from build123d import *

# Parameters (mm, degrees)
ESBO_O1_R                = 5.25
ESBO_O1_R_2              = 3.225
ESBO_O1_R_3              = 2.5
RESSALTO_EXTRUS_O1_DEPTH = 5


with BuildPart() as part:
    # Esboço1 → Ressalto-extrusão1 (new body)
    with BuildSketch(Plane.XY):
        with BuildLine():
            Line((0.238095238, -10.714285714), (31.238095238, -10.714285714))
            ThreePointArc((31.238095238, -10.714285714), (34.066522363, -11.88585859), (35.238095238, -14.714285714))
            Line((35.238095238, -14.714285714), (35.238095238, -18.714285714))
            ThreePointArc((35.238095238, -18.714285714), (35.823881676, -20.128499277), (37.238095238, -20.714285714))
            Line((37.238095238, -20.714285714), (53.238095238, -20.714285714))
            ThreePointArc((53.238095238, -20.714285714), (54.6523088, -20.128499277), (55.238095238, -18.714285714))
            Line((55.238095238, -18.714285714), (55.238095238, -2.714285714))
            ThreePointArc((55.238095238, -2.714285714), (54.6523088, -1.300072152), (53.238095238, -0.714285714))
            Line((53.238095238, -0.714285714), (31.847818571, -0.714285714))
            ThreePointArc((31.847818571, -0.714285714), (14.124879647, 4.104636838), (1.282253299, 17.234432234))
            ThreePointArc((1.282253299, 17.234432234), (-0.185475427, 18.73498028), (-2.210954161, 19.285714286))
            Line((-2.210954161, 19.285714286), (-17.761904762, 19.285714286))
            ThreePointArc((-17.761904762, 19.285714286), (-19.176118324, 19.871500723), (-19.761904762, 21.285714286))
            Line((-19.761904762, 21.285714286), (-19.761904762, 27.285714286))
            ThreePointArc((-19.761904762, 27.285714286), (-20.3476912, 28.699927848), (-21.761904762, 29.285714286))
            Line((-21.761904762, 29.285714286), (-37.761904762, 29.285714286))
            ThreePointArc((-37.761904762, 29.285714286), (-39.176118324, 28.699927848), (-39.761904762, 27.285714286))
            Line((-39.761904762, 27.285714286), (-39.761904762, -18.714285714))
            ThreePointArc((-39.761904762, -18.714285714), (-39.176118324, -20.128499277), (-37.761904762, -20.714285714))
            Line((-37.761904762, -20.714285714), (-21.761904762, -20.714285714))
            ThreePointArc((-21.761904762, -20.714285714), (-20.3476912, -20.128499277), (-19.761904762, -18.714285714))
            Line((-19.761904762, -18.714285714), (-19.761904762, -14.714285714))
            ThreePointArc((-19.761904762, -14.714285714), (-18.590331887, -11.88585859), (-15.761904762, -10.714285714))
            Line((-15.761904762, -10.714285714), (0.238095238, -10.714285714))
        make_face()
        with Locations((-29.761904762, -13.571428571)):
            Circle(ESBO_O1_R, mode=Mode.SUBTRACT)
        with Locations((-29.761904762, 21.904761905)):
            Circle(ESBO_O1_R_2, mode=Mode.SUBTRACT)
        with Locations((-4.761904762, 4.285714286)):
            Circle(ESBO_O1_R_3, mode=Mode.SUBTRACT)
        with Locations((45.476190476, -10.714285714)):
            Circle(ESBO_O1_R, mode=Mode.SUBTRACT)
    extrude(amount=RESSALTO_EXTRUS_O1_DEPTH)


solid = part.part
Could you check a few things on this model? Use its own coordinates, in mm. A direction names the side the tool comes from. Give positions to 0.01 mm unless a question says otherwise; leave off trailing zeros. Loops run counter-clockwise (first coordinate to the right, second up) from the corner with the lowest first, then second, coordinate; pieces in that order, holes last. Notation, with made-up numbers: (11.25, 16) -> (18.25, 16) arc R13 cw to (18.25, 31) -> close; hole circle Ø4 at (86.5, 2). An arc over 180 degrees is marked (long way). Return JSON: item names as keys, results as strings.
Item 1: I need wall thicknesses on L1, parallel to X at y = -18, z = 3; L2, parallel to Y at x = 45, z = 4.15; L3, parallel to X at y = -17.5, z = 3.15. Which ranges of each line are inside material? Lowest first, please. Write a range as from..to.
Geometry results:
{"L1": "x = -39.76..-32.58, -26.94..-19.76, 35.24..55.24", "L2": "y = -20.71..-15.94, -5.49..-0.71", "L3": "x = -39.76..-33.24, -26.28..-19.76, 35.24..55.24"}
Item 2: I'm going to push flat-ended pins straight in: pin 1 (2.5 mm diameter, centred on y = 25, z = 3.5, fed in from +X); pin 2 (1.5 mm diameter, centred on x = 41, z = 1.5, fed in from +Y); pin 3 (2.5 mm diameter, centred on x = -12, z = 1.5, fed in from +Y). Where does each tip first touch, or does it pass through?
Geometry results:
{"pin 1": "stops at x = -19.76", "pin 2": "stops at y = -0.71", "pin 3": "stops at y = 19.29"}
Item 3: If we section it at A-A on x = 43: List the corners of the cut face in (y, z) for me.
Geometry results:
{"outline": "(-20.71, 0) -> (-15.34, 0) -> (-15.34, 5) -> (-20.71, 5) -> close; (-6.08, 0) -> (-0.71, 0) -> (-0.71, 5) -> (-6.08, 5) -> close"}
Item 4: Which directions (+Z, -Z, +X, -X, +Y, -Y) give clear straight access to the entire face, cutting with the end or side of a thin tool? Please do faces 1 (the cylindrical face through (35.808, -20.113, 2.465)), 2 (the flat face through (-39.762, 5, 2)), 3 (the flat face through (43, -0.714, 2)).
Geometry results:
{"face 1": "+Z, -Z, -Y", "face 2": "+Z, -Z, -X, +Y, -Y", "face 3": "+Z, -Z, +X, +Y"}
Item 5: If we section it at D-D on x = -12.5: List the corners of the cut face in (y, z) for me, plus the area to 3 significant figures.
Geometry results:
{"outline": "(-10.71, 0) -> (19.29, 0) -> (19.29, 5) -> (-10.71, 5) -> close", "area": "150 mm²"}
Item 6: If we section it at B-B on y = 24: List the corners of the cut face in (x, z) for me, plus the area to 3 significant figures.
Geometry results:
{"outline": "(-39.76, 0) -> (-32.21, 0) -> (-32.21, 5) -> (-39.76, 5) -> close; (-27.31, 0) -> (-19.76, 0) -> (-19.76, 5) -> (-27.31, 5) -> close", "area": "75.5 mm²"}
Item 7: We'd pull the mould along X, two halves only. Please class faces 4 (the cylindrical face through (-39.192, -20.113, 2.465)), 5 (the cylindrical face through (54.64, -20.14, 2.46)), 6 (the flat face through (-3, -1, 0)), 7 (the cylindrical face through (-33.9, -16.8, 2.5)): +X half, -X half, draft (parallel to the pull), parting line (faces both ways), or undercut.
Geometry results:
{"face 4": "-X half", "face 5": "+X half", "face 6": "draft", "face 7": "undercut"}
Item 8: If we section it at C-C on z = 2.2: List the corners of the cut face in (x, y) for me (3 decimals).
Geometry results:
{"outline": "(-39.762, -18.714) arc R2 ccw to (-37.762, -20.714) -> (-21.762, -20.714) arc R2 ccw to (-19.762, -18.714) -> (-19.762, -14.714) arc R4 cw to (-15.762, -10.714) -> (31.238, -10.714) arc R4 cw to (35.238, -14.714) -> (35.238, -18.714) arc R2 ccw to (37.238, -20.714) -> (53.238, -20.714) arc R2 ccw to (55.238, -18.714) -> (55.238, -2.714) arc R2 ccw to (53.238, -0.714) -> (31.848, -0.714) arc R35 cw to (1.282, 17.234) arc R4 ccw to (-2.211, 19.286) -> (-17.762, 19.286) arc R2 cw to (-19.762, 21.286) -> (-19.762, 27.286) arc R2 ccw to (-21.762, 29.286) -> (-37.762, 29.286) arc R2 ccw to (-39.762, 27.286) -> close; hole circle Ø10.5 at (-29.762, -13.571); hole circle Ø6.45 at (-29.762, 21.905); hole circle Ø5 at (-4.762, 4.286); hole circle Ø10.5 at (45.476, -10.714)"}
